from build123d import *

# Parameters (mm, degrees)
F0_R     = 2.75
F0_R_2   = 11
F0_R_3   = 9.25
F1_DEPTH = 6
F0_R_4   = 2
F0_W     = 123
F0_H     = 56
F2_DEPTH = 3.5
F0_R_5   = 9.125
F3_DEPTH = 3
F0_R_6   = 8
F4_DEPTH = 4.5


with BuildPart() as f1:
    # F0 (on Top) → F1 (new body)
    with BuildSketch(Plane.XY):
        with BuildLine():
            Line((41.75, -57), (101, -57))
            ThreePointArc((101, -57), (102.414214, -56.414214), (103, -55))
            Line((103, -55), (103, 55))
            ThreePointArc((103, 55), (102.414214, 56.414214), (101, 57))
            Line((101, 57), (-101, 57))
            ThreePointArc((-101, 57), (-102.414214, 56.414214), (-103, 55))
            Line((-103, 55), (-103, -55))
            ThreePointArc((-103, -55), (-102.414214, -56.414214), (-101, -57))
            Line((-101, -57), (-41.75, -57))
            Line((-41.75, -57), (-35.25, -57))
            Line((-35.25, -57), (0, -57))
            Line((0, -57), (35.25, -57))
            Line((35.25, -57), (41.75, -57))
        make_face()
        with BuildLine():
            ThreePointArc((70, -39.375), (69.414214, -40.789214), (68, -41.375))
            Line((68, -41.375), (-68, -41.375))
            ThreePointArc((-68, -41.375), (-69.414214, -40.789214), (-70, -39.375))
            Line((-70, -39.375), (-70, 19.375))
            ThreePointArc((-70, 19.375), (-69.414214, 20.789214), (-68, 21.375))
            Line((-68, 21.375), (68, 21.375))
            ThreePointArc((68, 21.375), (69.414214, 20.789214), (70, 19.375))
            Line((70, 19.375), (70, -39.375))
        make_face(mode=Mode.SUBTRACT)
        with Locations((-93.5, 25)):
            Circle(F0_R, mode=Mode.SUBTRACT)
        with Locations((-61.5, 39)):
            Circle(F0_R_2, mode=Mode.SUBTRACT)
        with Locations((-35.5, 39)):
            Circle(F0_R_3, mode=Mode.SUBTRACT)
        with Locations((93.5, 25)):
            Circle(F0_R, mode=Mode.SUBTRACT)
        with BuildLine():
            Line((-35.25, -59), (-35.25, -57))
            Line((-35.25, -57), (-41.75, -57))
            Line((-41.75, -57), (-41.75, -59))
            ThreePointArc((-41.75, -59), (-41.457107, -59.707107), (-40.75, -60))
            Line((-40.75, -60), (-36.25, -60))
            ThreePointArc((-36.25, -60), (-35.542893, -59.707107), (-35.25, -59))
        make_face()
        with BuildLine():
            Line((41.75, -59), (41.75, -57))
            Line((41.75, -57), (35.25, -57))
            Line((35.25, -57), (35.25, -59))
            ThreePointArc((35.25, -59), (35.542893, -59.707107), (36.25, -60))
            Line((36.25, -60), (40.75, -60))
            ThreePointArc((40.75, -60), (41.457107, -59.707107), (41.75, -59))
        make_face()
    extrude(amount=F1_DEPTH)

    # F0 (on Top) → F2 (join)
    with BuildSketch(Plane.XY):
        with BuildLine():
            Line((-68, -41.375), (68, -41.375))
            ThreePointArc((68, -41.375), (69.414214, -40.789214), (70, -39.375))
            Line((70, -39.375), (70, 19.375))
            ThreePointArc((70, 19.375), (69.414214, 20.789214), (68, 21.375))
            Line((68, 21.375), (-68, 21.375))
            ThreePointArc((-68, 21.375), (-69.414214, 20.789214), (-70, 19.375))
            Line((-70, 19.375), (-70, -39.375))
            ThreePointArc((-70, -39.375), (-69.414214, -40.789214), (-68, -41.375))
        make_face()
        with Locations((-66, -37.625)):
            Circle(F0_R_4, mode=Mode.SUBTRACT)
        with Locations((0, -10)):
            Rectangle(F0_W, F0_H, mode=Mode.SUBTRACT)
        with Locations((66, -37.625)):
            Circle(F0_R_4, mode=Mode.SUBTRACT)
        with Locations((-66, 17.625)):
            Circle(F0_R_4, mode=Mode.SUBTRACT)
        with Locations((66, 17.625)):
            Circle(F0_R_4, mode=Mode.SUBTRACT)
    extrude(amount=F2_DEPTH)

    # F0 (on Top) → F3 (join)
    with BuildSketch(Plane.XY):
        with Locations((-61.5, 39)):
            Circle(F0_R_2)
        with Locations((-61.5, 39)):
            Circle(F0_R_5, mode=Mode.SUBTRACT)
    extrude(amount=F3_DEPTH)

    # F0 (on Top) → F4 (join)
    with BuildSketch(Plane.XY):
        with Locations((-35.5, 39)):
            Circle(F0_R_3)
        with Locations((-35.5, 39)):
            Circle(F0_R_6, mode=Mode.SUBTRACT)
    extrude(amount=F4_DEPTH)


solid = f1.part
Model file for the job. Use its own axes, mm. A direction names the side the tool comes from. Give positions to 0.01 mm unless a question says otherwise; leave off trailing zeros. Loops run counter-clockwise (first coordinate to the right, second up) from the corner with the lowest first, then second, coordinate; pieces in that order, holes last. Notation, with made-up numbers: (22.5, 66.5) - (53.5, 66.5) arc R28 ccw to (53.5, 103.5) - close; hole circle Ø8 at (-12, 38). An arc over 180 degrees is marked (long way). Use one line per item in the form item = value.
(1) 3-axis set-ups, long thin cutter, end or side, ignore diameter. For faces 1 (the face through (-72, -57, 3)), 2 (the face through (0, -57, 3)), 3 (the face through (-70, 43, 3)): which of +Z, -Z, +X, -X, +Y, -Y reach the whole face in a straight line?
Determined:
face_1 = +Z, -Z, -X, -Y
face_2 = +Z, -Z, -Y
face_3 = +Z
(2) Cut at C-C (y = 5). Give the cut face in (x, z), then the cut area to 4 significant figures.
Determined:
outline = (-103, 0) - (-61.5, 0) - (-61.5, 3.5) - (-70, 3.5) - (-70, 6) - (-103, 6) - close; (61.5, 0) - (103, 0) - (103, 6) - (70, 6) - (70, 3.5) - (61.5, 3.5) - close
area = 455.5 mm^2
(3) Drill centre lines: L1, parallel to Y at x = -15.5, z = 3.4; L2, parallel to X at y = 7.5, z = 4.8; L3, parallel to X at y = 44.5, z = 2.2. Where is each one in solid material? Low to high.
Determined:
L1 = -57 to -38, 18 to 57
L2 = -103 to -70, 70 to 103
L3 = -103 to -68.78, -54.22 to -41.31, -29.69 to 103
(4) Cut at D-D (z = 1.6). Count the separate pieces of the cut face and the enclosed holes in it, then the cut area to 3 significant figures.
Determined:
separate_pieces = 1
enclosed_holes = 9
area = 16,100 mm^2
(5) Drop flat-ended pins along their axis: P1, Ø1.8, axis at x = -60.5, z = 4.5, coming from the -Y side; P2, Ø3.5, axis at x = -93.5, y = 25, coming from the +Z side; P3, Ø1.6, axis at y = -58, z = 3.5, coming from the +X side. Give the stop position or say it passes through.
Determined:
P1 = -57
P2 = through
P3 = 41.75
(6) Pull direction X, two halves, no side cores. Call faces 4 (the face through (-69.61, 46.43, 4.48)), 5 (the face through (65.57, -39.58, 1.73)), 6 (the face through (-103, 1, 3)), 7 (the face through (71, -57, 3)): pulls with the +X half, pulls with the -X half, needs draft (parallel to the pull), parting line crosses it, or undercut.
Determined:
face_4 = undercut
face_5 = undercut
face_6 = pulls with the -X half
face_7 = needs draft
(7) Cut at B-B (y = 25). Give the cut face in (x, z), then the cut area to 3 significant figures.
Determined:
outline = (-103, 0) - (-96.25, 0) - (-96.25, 6) - (-103, 6) - close; (-90.75, 0) - (90.75, 0) - (90.75, 6) - (-90.75, 6) - close; (96.25, 0) - (103, 0) - (103, 6) - (96.25, 6) - close
area = 1,170 mm^2
(8) Cut at A-A (x = -21.5). Give the cut face in (y, z) (3 decimals), then the cut area to 3 significant figures.
Determined:
outline = (-57, 0) - (-38, 0) - (-38, 3.5) - (-41.375, 3.5) - (-41.375, 6) - (-57, 6) - close; (18, 0) - (57, 0) - (57, 6) - (21.375, 6) - (21.375, 3.5) - (18, 3.5) - close
area = 331 mm^2
